```python
from build123d import *

# Parameters (mm, degrees)
F0_R     = 30
F0_R_2   = 2.5
F1_DEPTH = 14.9
F2_R     = 3.2
F3_R     = 15.1
F4_DEPTH = 14.6
F5_R     = 3.2
F6_R     = 7.3
F7_DEPTH = 60


with BuildPart() as f1:
    # F0 (on Top) → F1 (new body)
    with BuildSketch(Plane.XY):
        Circle(F0_R)
        with Locations((0, -22.3)):
            Circle(F0_R_2, mode=Mode.SUBTRACT)
        with Locations((-22.3, 0)):
            Circle(F0_R_2, mode=Mode.SUBTRACT)
        with Locations((22.3, 0)):
            Circle(F0_R_2, mode=Mode.SUBTRACT)
        with Locations((0, 22.3)):
            Circle(F0_R_2, mode=Mode.SUBTRACT)
    extrude(amount=F1_DEPTH)

    # F2
    f2_edges = [f1.edges().sort_by_distance(p)[0] for p in [
        (-30, 0, 14.9),
    ]]
    fillet(f2_edges, radius=F2_R)

    # F3 (on face) → F4 (join)
    with BuildSketch(Plane.XY.offset(14.9)):
        Circle(F3_R)
    extrude(amount=F4_DEPTH)

    # F5
    f5_edges = [f1.edges().sort_by_distance(p)[0] for p in [
        (-15.1, 0, 29.5),
    ]]
    fillet(f5_edges, radius=F5_R)

    # F6 (on face) → F7 (cut)
    with BuildSketch(Plane.XY.offset(29.5)):
        Circle(F6_R)
    extrude(amount=-F7_DEPTH, mode=Mode.SUBTRACT)


solid = f1.part
```
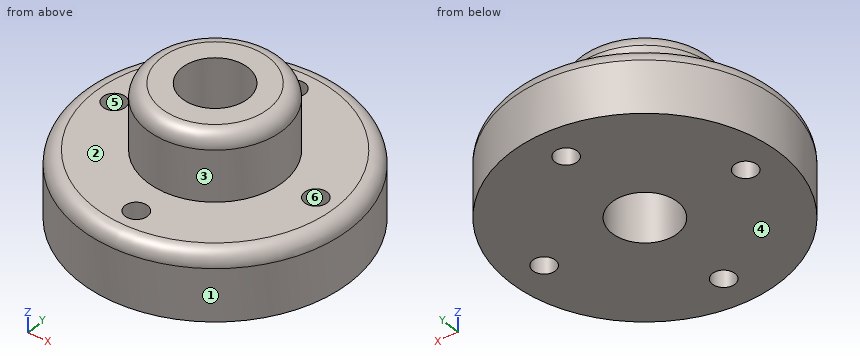
Can you work these out from the model? Positions are in its coordinate system, mm. Face numbers are marked on the shaded views. A direction names the side the tool comes from. Give positions to 0.01 mm unless a question says otherwise; leave off trailing zeros. Order: outer loops, then holes, each group sorted by start corner. A loop starts at its lowest first (then second) coordinate and runs counter-clockwise, first axis right, second up. Notation, with made-up numbers: M 85,-32.75 L 121,-32.75 A28 cw 121,5.25 Z; hole C -32.5,3.5 d4. An arc over 180 degrees is marked long. Write item = value, one per line. Start each with the question number.
Q1. Suppose I cut it at B-B (z = 10.75). Write out the boundary of the cut face in (x, y).
Q2. I need wall thicknesses on probe 1 along Y at (x, z) = (0, 9.75); probe 2 along Y at (x, z) = (0, 12.25); probe 3 along Y at (x, z) = (0, 15.5). Which ranges of each line are inside material? Lowest first, please. Write a range as [from, to].
Q3. Suppose I cut it at C-C (z = 25.5). Write out the boundary of the cut face in (x, y).
Q4. Will these pins go through, and if not, where does the flat tip stop? pin 1 Ø6 at (x, z) = (-10, 11) entering from -Y; pin 2 Ø6 at (y, z) = (-3.5, 20) entering from -X; pin 3 Ø3 at (y, z) = (-16, 5.5) entering from -X.
Q5. We'd pull the mould along Y, two halves only. Please class the marked faces 3, 4, 5 and 6: pulls with the +Y half, pulls with the -Y half, needs draft (parallel to the pull), parting line crosses it, or undercut.
Q6. For the marked faces 1 and 2, which set-ups out of +Z, -Z, +X, -X, +Y, -Y let a thin tool reach every point of the face, with its end or its side?
Q7. Suppose I cut it at A-A (x = 0). Write out the boundary of the cut face in (y, z).
Check result:
q1.outline = C 0,0 d60; hole C -22.3,0 d5; hole C 0,0 d14.6; hole C 0,-22.3 d5; hole C 0,22.3 d5; hole C 22.3,0 d5
q2.probe_1 = [-30, -24.8], [-19.8, -7.3], [7.3, 19.8], [24.8, 30]
q2.probe_2 = [-29.95, -24.8], [-19.8, -7.3], [7.3, 19.8], [24.8, 29.95]
q2.probe_3 = [-15.1, -7.3], [7.3, 15.1]
q3.outline = C 0,0 d30.2; hole C 0,0 d14.6
q4.pin_1 = -29.17
q4.pin_2 = -15.09
q4.pin_3 = -26.26
q5.face_3 = parting line crosses it
q5.face_4 = needs draft
q5.face_5 = undercut
q5.face_6 = undercut
q6.face_1 = +Z, -Z
q6.face_2 = +Z
q7.outline = M -30,0 L -24.8,0 L -24.8,14.9 L -26.8,14.9 A3.2 ccw -30,11.7 Z; M -19.8,0 L -7.3,0 L -7.3,29.5 L -11.9,29.5 A3.2 ccw -15.1,26.3 L -15.1,14.9 L -19.8,14.9 Z; M 7.3,0 L 19.8,0 L 19.8,14.9 L 15.1,14.9 L 15.1,26.3 A3.2 ccw 11.9,29.5 L 7.3,29.5 Z; M 24.8,0 L 30,0 L 30,11.7 A3.2 ccw 26.8,14.9 L 24.8,14.9 Z
